Can you work these out from the model? Positions are in its coordinate system, mm. Face numbers are marked on the shaded views. A direction names the side the tool comes from. Give positions to 0.01 mm unless a question says otherwise; leave off trailing zeros. Write each loop counter-clockwise with the first axis right and the second up, starting at its lowest first coordinate (ties: lowest second). Pieces come first, ordered by that corner, then holes.
from build123d import *

# Parameters (mm, degrees)
SKETCH2_R           = 5
SKETCH2_R_2         = 2.75
BOSS_EXTRUDE1_DEPTH = 6
BOSS_EXTRUDE2_DEPTH = 3
FILLET1_R           = 2
FILLET2_R           = 5


with BuildPart() as part:
    # Sketch2 → Boss-Extrude1 (new body)
    # profile 1 of 2: a face of its own
    with BuildSketch(Plane.XY):
        with Locations((0, 27.75)):
            Circle(SKETCH2_R)
        with Locations((0, 27.75)):
            Circle(SKETCH2_R_2, mode=Mode.SUBTRACT)
    # profile 2 of 2: a face of its own
    with BuildSketch(Plane.XY):
        with BuildLine():
            ThreePointArc((5, 27.75), (0, 22.75), (-5, 27.75))
            Line((-5, 27.75), (-5, 19.75))
            Line((-5, 19.75), (5, 19.75))
            Line((5, 19.75), (5, 27.75))
        make_face()
    extrude(amount=BOSS_EXTRUDE1_DEPTH)

    # Sketch3 → Boss-Extrude2 (add)
    with BuildSketch(Plane.XY.offset(3)):
        with BuildLine():
            Line((5, 19.75), (-5, 19.75))
            Line((-5, 19.75), (-13.753194099, 19.75))
            Line((-13.753194099, 19.75), (-13.753194099, 14.75))
            Line((-13.753194099, 14.75), (-20.753194099, 14.75))
            Line((-20.753194099, 14.75), (-20.753194099, 11.59876127))
            Line((-20.753194099, 11.59876127), (-14.900453075, 11.59876127))
            Line((-14.900453075, 11.59876127), (-8.795188245, 11.59876127))
            ThreePointArc((-8.795188245, 11.59876127), (0, 14.556325061), (8.795188245, 11.59876127))
            Line((8.795188245, 11.59876127), (20.753194099, 11.59876127))
            Line((20.753194099, 11.59876127), (20.753194099, 14.75))
            Line((20.753194099, 14.75), (13.753194099, 14.75))
            Line((13.753194099, 14.75), (13.753194099, 19.75))
            Line((13.753194099, 19.75), (5, 19.75))
        make_face()
    extrude(amount=BOSS_EXTRUDE2_DEPTH)

    # Fillet1
    fillet1_edges = [part.edges().sort_by_distance(p)[0] for p in [
        (5, 19.75, 4.5),
        (-5, 19.75, 4.5),
        (-20.753194099, 11.59876127, 4.5),
        (20.753194099, 11.59876127, 4.5),
        (13.753194099, 19.75, 4.5),
        (-13.753194099, 19.75, 4.5),
    ]]
    fillet(fillet1_edges, radius=FILLET1_R)

    # Fillet2
    fillet2_edges = [part.edges().sort_by_distance(p)[0] for p in [
        (-8.795188245, 11.59876127, 4.5),
        (8.795188245, 11.59876127, 4.5),
    ]]
    fillet(fillet2_edges, radius=FILLET2_R)


solid = part.part
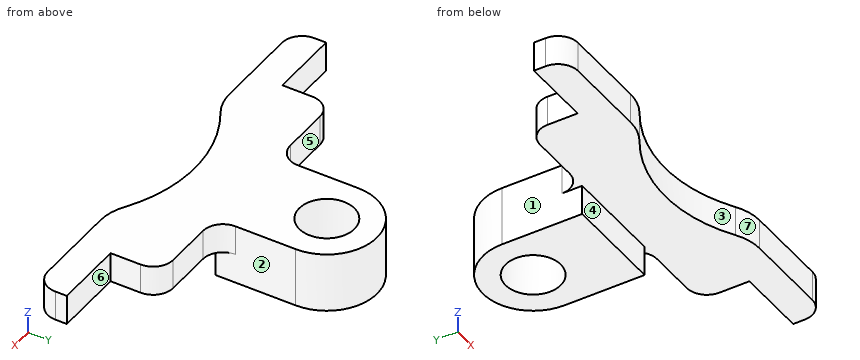
(1) Imagine slicing it at A-A, the plane z = 4.95. Write out the boundary of the cut face in (x, y).
Returned:
outline: (-20.75, 13.6) arc R2 ccw to (-18.75, 11.6) - (-10.34, 11.6) arc R5 ccw to (-7.7, 12.35) arc R14.56 cw to (7.7, 12.35) arc R5 ccw to (10.34, 11.6) - (18.75, 11.6) arc R2 ccw to (20.75, 13.6) - (20.75, 14.75) - (13.75, 14.75) - (13.75, 17.75) arc R2 ccw to (11.75, 19.75) - (7, 19.75) arc R2 cw to (5, 21.75) - (5, 27.75) arc R5 ccw to (-5, 27.75) - (-5, 21.75) arc R2 cw to (-7, 19.75) - (-11.75, 19.75) arc R2 ccw to (-13.75, 17.75) - (-13.75, 14.75) - (-20.75, 14.75) - close; hole circle Ø5.5 at (0, 27.75)
(2) Imagine slicing it at B-B, the plane x = 0. Write out the boundary of the cut face in (y, z).
Returned:
outline: (14.56, 3) - (19.75, 3) - (19.75, 0) - (25, 0) - (25, 6) - (14.56, 6) - close; (30.5, 0) - (32.75, 0) - (32.75, 6) - (30.5, 6) - close
(3) For the marked faces 4, 5, 6 and 7, which set-ups out of +Z, -Z, +X, -X, +Y, -Y let a thin tool reach every point of the face, with its end or its side?
Returned:
face 4: -Z, +X, -X, -Y
face 5: +Z, -Z, -X, +Y
face 6: +Z, -Z, +X, +Y
face 7: +Z, -Z, -Y
(4) Will these pins go through, and if not, where does the flat tip stop? P1, Ø2, axis at y = 15.5, z = 2.5, coming from the -X side; P2, Ø2, axis at y = 21, z = 4, coming from the -X side; P3, Ø2.5, axis at x = 16.5, z = 4.5, coming from the +Y side; P4, Ø1.5, axis at y = 17, z = 4, coming from the -X side.
Returned:
P1: stops at x = -20.75
P2: stops at x = -6.03
P3: stops at y = 14.75
P4: stops at x = -13.75
(5) If I drill on L1, parallel to Y at x = 0, z = 3.3; L2, parallel to Y at x = 0, z = 2.35; L3, parallel to X at y = 23, z = 3.6, over which ranges is the centre line in solid material (lowest first)?
Returned:
L1: y = 14.56 to 25, 30.5 to 32.75
L2: y = 19.75 to 25, 30.5 to 32.75
L3: x = -5 to 5
(6) Imagine slicing it at D-D, the plane x = 18. Write out the boundary of the cut face in (y, z), plus the area to 3 significant figures.
Returned:
outline: (11.6, 3) - (14.75, 3) - (14.75, 6) - (11.6, 6) - close
area: 9.45 mm2
(7) Imagine slicing it at C-C, the plane y = 29.25. Write out the boundary of the cut face in (x, z), plus the area to 3 significant figures.
Returned:
outline: (-4.77, 0) - (-2.3, 0) - (-2.3, 6) - (-4.77, 6) - close; (2.3, 0) - (4.77, 0) - (4.77, 6) - (2.3, 6) - close
area: 29.6 mm2
(8) If we mould it in two halves opening along X, with no side actions, what happens to the marked faces 1, 2 and 3? For each: +X half, -X half, draft (parallel to the pull), parting line (faces both ways), or undercut.
Returned:
face 1: -X half
face 2: +X half
face 3: undercut
